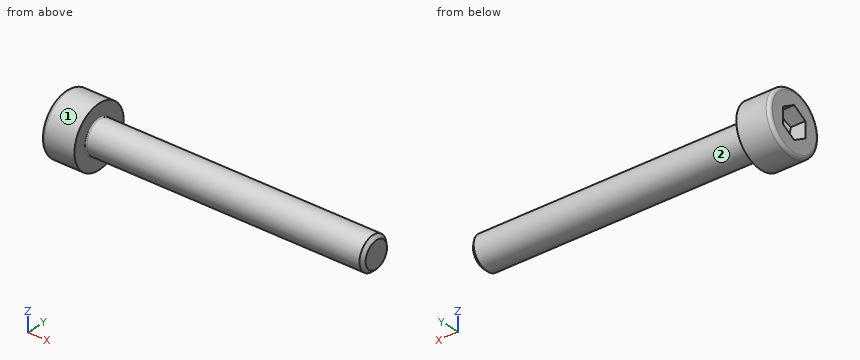
Autodesk Inventor part; units mm, degrees
ref_plane "Work Plane1" through (29, 0, 0) normal (0, -1, 0) x (1, 0, 0)
ref_plane "YZ Plane" through (0, 0, 0) normal (1, 0, 0) x (0, 1, 0)
ref_plane "XZ Plane" through (0, 0, 0) normal (0, 1, 0) x (-1, 0, 0)
sketch "Sketch1" plane through (0, 0, 0) normal (0, 0, 1) x (1, 0, 0)
  line L0 (-0.8667, 0) -> (25, 0)
  line L1 (25, 0) -> (25, 1.5)
  line L2 (25, 1.5) -> (18.25, 1.5)
  line L3 (18.25, 1.5) -> (17.9432, 1.5)
  line L4 (17.9432, 1.5) -> (0, 1.5)
  line L5 (0, 1.5) -> (0, 2.75)
  line L6 (0, 2.75) -> (-3, 2.75)
  line L7 (-3, 2.75) -> (-3, 1.4434)
  line L8 (-3, 1.4434) -> (-1.7, 1.4434)
  line L9 (-1.7, 1.4434) -> (-0.8667, 0)
  line L10 (-8.6, 0) -> (30.6, 0)
  line L11 (0, -0.55) -> (0, 3.3)
  line L12 (18.25, 1.5) -> (0, 1.5) construction
  dimension "d1" = 6.75
  dimension "d2" = 0.3068
  dimension "d3" = 3
  dimension "d4" = 1.3
  dimension "d5" = 60
  dimension "d6" = 3
  dimension "d7" = 3
  dimension "d8" = 2.8868
  dimension "d9" = 5.5
  dimension "d26" = 25
revolve "Body" add sketch "Sketch1" angle 360 about axis through (-0.8667, 0, 0) along (1, 0, 0)
sketch "Sketch2" plane through (-3, 0, 0) normal (-1, 0, 0) x (0, 0, 1)
  circle A0 centre (0, 0) radius 1.4434
  line L0 (0, -3.85) -> (0, 3.85)
  line L1 (-3.85, 0) -> (3.85, 0)
  line L2 (1.4434, 0) -> (0.7217, -1.25)
  line L3 (0.7217, -1.25) -> (-0.7217, -1.25)
  line L4 (-0.7217, -1.25) -> (-1.4434, 0)
  line L5 (-1.4434, 0) -> (-0.7217, 1.25)
  line L6 (-0.7217, 1.25) -> (0.7217, 1.25)
  line L7 (0.7217, 1.25) -> (1.4434, 0)
extrude "Slot" add sketch "Sketch2" against normal up to next contours L7 A0 | A0 L2 | L6 L0 A0 | A0 L0 L3 | L0 L6 A0 | A0 L3 L0 | L4 A0 | A0 L5
fillet "Fillet1" radius 0.3 1 edges at (-3, -2.75, 0)
thread "Thread"
chamfer "Chamfer1" distance 0.3067 distance2 0.3067 1 edges at (25, -1.5, 0) measured on face at (25, 0.2885, 0.9187)
ref_plane "Work Plane1" through (29, 0, 0) normal (0, -1, 0) x (1, 0, 0)
fillet "Fillet2" radius 0.1 1 edges at (0, -1.5, 0)
equation "\"d1\" = GEL"
equation "\"d3\" = KOH"
equation "\"d4\" = INTI"
equation "\"d6\" = GD"
equation "\"d7\" = BDM"
equation "\"d8\" = 1.1547 * SW"
equation "\"d9\" = KOD"
equation "\"d17\" = RR"
equation "\"d13\" = GEL"
equation "\"d15\" = -0.5 * SPD + 0.5 * GD"
equation "\"d16\" = GUL"
equation "\"d30\" = R"
equation "\"GD\" = NND"
equation "\"NLG\" = 8"
equation "\"GEL\" = 6.75"
equation "\"KOD\" = 5.5"
equation "\"KOH\" = NND"
equation "\"INTI\" = 1.3"
equation "\"GAL\" = 0.61345 * PTC"
equation "\"GUL\" = 0.61345 * PTC"
equation "\"BDM\" = NND"
equation "\"SW\" = 2.5"
equation "\"RR\" = 0.1 * NND"
equation "\"SPD\" = NND - 1.2269 * PTC"
equation "\"R\" = 0.1"
equation "\"PHH\" = 0.13"
equation "\"GD1\" = THREADDIA - 1.2269 * PTC"
equation "\"THREADDIA\" = 3"
equation "\"FAWI\" = 45deg"
equation "\"PTC\" = 0.5"
equation "\"KOH1\" = 2.7"
equation "\"NND\" = 3"
equation "\"TOA\" = 30deg"
equation "\"E0\" = 1.155 * SW"
properties part number "AS 1420 - 1973 - M3 x 8" material "Steel, Mild"
For this review, take the finished solid that the model builds, in its own axes (mm). Face numbers are marked on the shaded views. A direction names the side the tool comes from. Coordinates: 2 decimals unless noted, no trailing zeros. Loops run counter-clockwise (first coordinate to the right, second up) from the corner with the lowest first, then second, coordinate; pieces in that order, holes last.
1. Insertion check: P1, Ø1.5, axis at x = 12.5, y = 2, coming from the +Z side; P2, Ø2, axis at x = 22, y = 1.5, coming from the +Z side; P3, Ø2, axis at x = 2.5, z = -2, coming from the +Y side. Each pin has a flat end and moves straight along its axis. Give the tip position at first contact, or say it passes through.
2. For the marked faces 1 and 2, list the 3-axis set-ups (+Z, -Z, +X, -X, +Y, -Y) from which the entire face can be reached by the end or side of a thin tool; tool diameter is ignored.
3. Add section A-A, the plane x = 5.25. Give the boundary of the cut face in (y, z), then the cut area to 3 significant figures.
4. For line 1 (X direction, y = 0, z = 1.9); line 2 (Z direction, x = 22.25, y = 0.9); line 3 (X direction, y = -0.5, z = -1.3), list the stretches that pass through material, from the lowest coordinate up.
Result:
1. P1: stops at z = 0.83
1. P2: stops at z = 1.41
1. P3: stops at y = 1.12
2. face 1: +X, -X
2. face 2: +X
3. outline: circle Ø3 at (0, 0)
3. area: 7.07 mm2
4. line 1: x = -3 to 0
4. line 2: z = -1.2 to 1.2
4. line 3: x = -3 to 24.8
